Check sheet for the modelled part. Datum: model origin and axes. Units: mm. Face numbers are marked on the shaded views. A direction names the side the tool comes from. Coordinates: 2 decimals unless noted, no trailing zeros. Order: outer loops, then holes, each group sorted by start corner. A loop starts at its lowest first (then second) coordinate and runs counter-clockwise, first axis right, second up.
1. Cross-section at D-D (y = 15). Enter the section's corners in (x, z), then the cut area to 3 significant figures.
2. Set-up check for the marked faces 1 and 2: record each of +Z, -Z, +X, -X, +Y, -Y from which the full face is reachable in a straight line by a thin tool's end or side.
3. Thickness scan on line 1 (Y direction, x = 0.95, z = 0); line 2 (Y direction, x = 8, z = 0); line 3 (X direction, y = 7.5, z = -4). Record the ranges inside material, lowest first.
4. Cross-section at A-A (x = 2.25). Enter the section's corners in (y, z).
5. Draft check along Y on the marked faces 3, 4 and 5. Enter one of: released by +Y, released by -Y, zero draft, split by the parting line, or undercut.
6. Cross-section at B-B (z = 0). Enter the section's corners in (x, y).
7. Cross-section at C-C (y = 12.5). Enter the section's corners in (x, z).
8. Gauge pin test, flat ends, axial feed: pin 1 Ø1.5 at (x, z) = (15, -4.5) entering from -Y; pin 2 Ø1 at (y, z) = (9.5, -8) entering from +X; pin 3 Ø3 at (y, z) = (3.5, 4) entering from +X; pin 4 Ø1.5 at (x, y) = (9.5, 13.5) entering from +Z. Record the tip position at first contact, or that the pin passes through.
```python
from build123d import *

# Parameters (mm, degrees)
BOSS_EXTRUDE1_DEPTH = 10
SKETCH2_R           = 3.57
CUT_EXTRUDE1_DEPTH  = 21
SKETCH3_R           = 5.5
CUT_EXTRUDE2_DEPTH  = 16.5


with BuildPart() as part:
    # Sketch1 → Boss-Extrude1 (new body, symmetric)
    with BuildSketch(Plane.XY):
        Polygon((0, 0), (0, 20), (20, 0), align=None)
    extrude(amount=BOSS_EXTRUDE1_DEPTH, both=True)

    # Sketch2 → Cut-Extrude1 (cut, through all)
    with BuildSketch(Plane(origin=(20, 0, 0), x_dir=(0, 0, -1), z_dir=(1, 0, 0))):
        with Locations((0, 10)):
            Circle(SKETCH2_R)
    extrude(amount=-CUT_EXTRUDE1_DEPTH, mode=Mode.SUBTRACT)

    # Sketch3 → Cut-Extrude2 (cut)
    with BuildSketch(Plane(origin=(20, 0, 0), x_dir=(0, 0, -1), z_dir=(1, 0, 0))):
        with Locations((0, 10)):
            Circle(SKETCH3_R)
    extrude(amount=-CUT_EXTRUDE2_DEPTH, mode=Mode.SUBTRACT)


solid = part.part
```
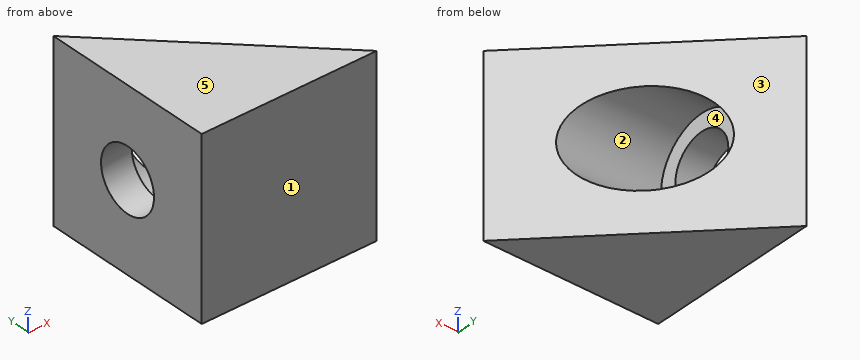
Data:
1. outline: (0, -10) - (5, -10) - (5, -2.29) - (3.5, -2.29) - (3.5, 2.29) - (5, 2.29) - (5, 10) - (0, 10) - close
1. area: 93.1 mm2
2. face 1: +Z, -Z, +X, -X, -Y
2. face 2: +X
3. line 1: y = 0 to 6.43, 13.57 to 19.05
3. line 2: y = 0 to 4.5
3. line 3: x = 0 to 3.5
4. outline: (0, -10) - (17.75, -10) - (17.75, 10) - (0, 10) - close; hole circle Ø7.14 at (10, 0)
5. face 3: released by +Y
5. face 4: undercut
5. face 5: zero draft
6. outline: (0, 0) - (20, 0) - (15.5, 4.5) - (3.5, 4.5) - (3.5, 6.43) - (0, 6.43) - close; (0, 13.57) - (3.5, 13.57) - (3.5, 15.5) - (4.5, 15.5) - (0, 20) - close
7. outline: (0, -10) - (7.5, -10) - (7.5, -4.9) - (3.5, -4.9) - (3.5, -2.55) - (0, -2.55) - close; (0, 2.55) - (3.5, 2.55) - (3.5, 4.9) - (7.5, 4.9) - (7.5, 10) - (0, 10) - close
8. pin 1: stops at y = 0
8. pin 2: stops at x = 11
8. pin 3: stops at x = 18
8. pin 4: passes through
